Part model, mm, in its own coordinate system. A direction names the side the tool comes from. Coordinates: 2 decimals unless noted, no trailing zeros. Write each loop counter-clockwise with the first axis right and the second up, starting at its lowest first coordinate (ties: lowest second). Pieces come first, ordered by that corner, then holes. Notation, with made-up numbers: (-16.75, 59.5) -> (-0.75, 59.5) arc R20 ccw to (-0.75, 75.5) -> close; hole circle Ø9 at (6, 8). An arc over 180 degrees is marked (long way). Write item = value, one per line.
from build123d import *

# Parameters (mm, degrees)
F1_DEPTH = 12.7


with BuildPart() as f1:
    # F0 (on Front) → F1 (new body)
    with BuildSketch(Plane.XZ):
        Polygon((-79.139665, 60.888402), (-74.736215, 60.888402), (-44.156749, 60.888402), (-44.156749, 88.708244), (-79.139665, 88.708244), align=None)
        Polygon((-102.624685, 63.956387), (-129.289985, 63.956387), (-129.289985, 27.619565), (-102.624685, 27.619565), (-102.624685, 31.707756), (-102.624685, 59.177574), align=None)
        Polygon((-73.513038, 40.182184), (-73.513038, 31.304672), (-73.513038, 13.690901), (-73.513038, 7.802445), (-44.156749, 7.802445), (-44.156749, 40.182184), (-51.251188, 40.182184), (-67.88642, 40.182184), align=None)
        Polygon((-73.513038, 31.304672), (-102.624685, 59.177574), (-102.624685, 31.707756), (-73.513038, 13.690901), align=None)
        Polygon((-74.736215, 60.888402), (-67.88642, 40.182184), (-51.251188, 40.182184), (-44.156749, 60.888402), align=None)
    extrude(amount=F1_DEPTH)


solid = f1.part
Q1. Mould opens along Z. For faces 5 (the face through (-48, -6, 40.182)), 6 (the face through (-61, -6, 88.708)), 7 (the face through (-79.14, -6, 75)) say: released by +Z, released by -Z, zero draft, split by the parting line, or undercut.
Model answer:
face_5 = undercut
face_6 = released by +Z
face_7 = zero draft
Q2. Saw through at D-D on z = 34.5. Give the cut face in (x, y).
Model answer:
outline = (-129.29, -12.7) -> (-76.85, -12.7) -> (-76.85, 0) -> (-129.29, 0) -> close; (-73.51, -12.7) -> (-44.16, -12.7) -> (-44.16, 0) -> (-73.51, 0) -> close
Q3. Probe line 1 (X direction, y = -11.5, z = 45); line 2 (X direction, y = -7.5, z = 63); line 3 (X direction, y = -4.25, z = 81). List the from-to ranges inside material, lowest first. Write a range as from..to.
Model answer:
line_1 = -129.29..-87.82, -69.48..-49.6
line_2 = -129.29..-102.62, -79.14..-44.16
line_3 = -79.14..-44.16
Q4. Pin check, flat tips, straight feed: pin 1 (1.3 mm diameter, centred on x = -78, y = -6.5, fed in from -Z); pin 2 (4.5 mm diameter, centred on y = -3.5, z = 11, fed in from -X); pin 3 (4 mm diameter, centred on x = -98, y = -7, fed in from +Z). Stop position of each tip, or through.
Model answer:
pin_1 = 16.07
pin_2 = -73.51
pin_3 = 56.66
Q5. Saw through at A-A on y = -1. Give the cut face in (x, z).
Model answer:
outline = (-129.29, 27.62) -> (-102.62, 27.62) -> (-102.62, 31.71) -> (-73.51, 13.69) -> (-73.51, 7.8) -> (-44.16, 7.8) -> (-44.16, 40.18) -> (-51.25, 40.18) -> (-44.16, 60.89) -> (-44.16, 88.71) -> (-79.14, 88.71) -> (-79.14, 60.89) -> (-74.74, 60.89) -> (-67.89, 40.18) -> (-73.51, 40.18) -> (-73.51, 31.3) -> (-102.62, 59.18) -> (-102.62, 63.96) -> (-129.29, 63.96) -> close
Q6. Saw through at C-C on x = -112.5. Give the cut face in (y, z).
Model answer:
outline = (-12.7, 27.62) -> (0, 27.62) -> (0, 63.96) -> (-12.7, 63.96) -> close
Q7. Saw through at B-B on z = 56.5. Give the cut face in (x, y), and give its area (3 significant figures).
Model answer:
outline = (-129.29, -12.7) -> (-99.83, -12.7) -> (-99.83, 0) -> (-129.29, 0) -> close; (-73.28, -12.7) -> (-45.66, -12.7) -> (-45.66, 0) -> (-73.28, 0) -> close
area = 725 mm²
Q8. Which spindle directions (+Z, -Z, +X, -X, +Y, -Y) get a long thin tool onto all of the face, cutting with end or side? Do faces 1 (the face through (-47.754, -6.261, 50.39)), 2 (the face through (-73.513, -6, 11)), 3 (the face through (-88.273, -6.261, 22.825)), 4 (the face through (-77, -6, 60.888)). Say none if no direction does.
Model answer:
face_1 = +X, +Y, -Y
face_2 = -Z, -X, +Y, -Y
face_3 = -Z, +Y, -Y
face_4 = +Y, -Y
